Geometry check sheet. Reference: the model listing, model coordinates, mm. Face numbers are marked on the shaded views. A direction names the side the tool comes from. Round coordinates to 2 decimals unless told otherwise and drop trailing zeros. Order: outer loops, then holes, each group sorted by start corner. A loop starts at its lowest first (then second) coordinate and runs counter-clockwise, first axis right, second up.
(1) Set-up check for the marked faces 4, 5 and 6: record each of +Z, -Z, +X, -X, +Y, -Y from which the full face is reachable in a straight line by a thin tool's end or side.
(2) Thickness scan on L1, parallel to X at y = 16.5, z = 0.5; L2, parallel to Y at x = -12, z = 3 (3 decimals); L3, parallel to Y at x = 14, z = -3.5 (3 decimals). Record the ranges inside material, lowest first.
(3) Draft check along X on the marked faces 1, 2 and 3. Enter one of: pulls with the +X half, pulls with the -X half, needs draft (parallel to the pull), parting line crosses it, or undercut.
(4) Cross-section at C-C on z = -2.75. Enter the section's corners in (x, y) (3 decimals).
(5) Gauge pin test, flat ends, axial feed: P1, Ø5, axis at x = -12.5, y = 10.5, coming from the -Z side; P2, Ø3, axis at x = -1.5, z = -2, coming from the +Y side; P3, Ø4, axis at x = 14.5, z = 1, coming from the -Y side. Record the tip position at first contact, or that the pin passes through.
(6) Cross-section at A-A on z = 2. Enter the section's corners in (x, y) (3 decimals).
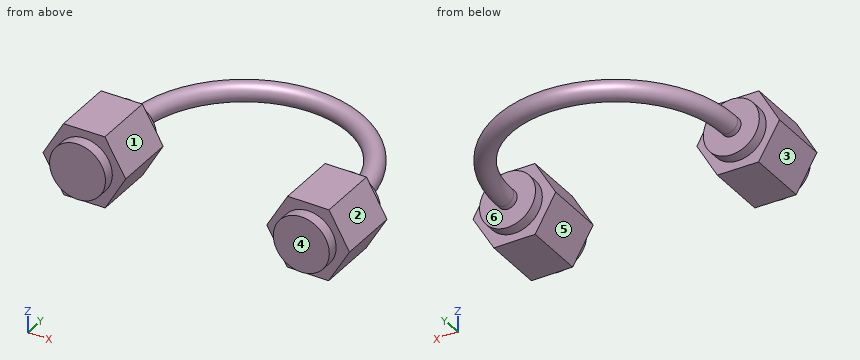
from build123d import *

# Parameters (mm, degrees)
SKETCH1_R             = 3.175
BOSS_EXTRUDE1_DEPTH   = 9.525
BOSS_EXTRUDE1_2_DEPTH = 9.525
BOSS_EXTRUDE2_START   = -1.27
BOSS_EXTRUDE2_DEPTH   = 6.985
SKETCH4_R             = 1.0922


with BuildPart() as part:
    # Sketch1 → Boss-Extrude1 (new body)
    with BuildSketch(Plane(origin=(0, 0, 0), x_dir=(1, 0, 0), z_dir=(0, 1, 0))):
        with Locations(Location((-12.7, 0, 0), (0, 0, 90))):
            Circle(SKETCH1_R)
    extrude(amount=BOSS_EXTRUDE1_DEPTH)

    # Sketch2 → Boss-Extrude2 (add)
    with BuildSketch(Plane(origin=(0, 9.525, 0), x_dir=(1, 0, 0), z_dir=(0, 1, 0)).offset(BOSS_EXTRUDE2_START)):
        Polygon((-8.007347217, -0.021706912), (-10.334874871, 4.053103065), (-15.027527654, 4.074809978), (-17.392652783, 0.021706912), (-15.065125129, -4.053103065), (-10.372472346, -4.074809978), align=None)
    boss_extrude2 = extrude(amount=-BOSS_EXTRUDE2_DEPTH)



with BuildPart() as body_2:
    # Sketch1 → Boss-Extrude1 2 (new body)
    with BuildSketch(Plane(origin=(0, 0, 0), x_dir=(1, 0, 0), z_dir=(0, 1, 0))):
        with Locations(Location((12.7, 0, 0), (0, 0, 90))):
            Circle(SKETCH1_R)
    extrude(amount=BOSS_EXTRUDE1_2_DEPTH)

    # Mirror1: Boss-Extrude2 across plane
    add(boss_extrude2.mirror(Plane(origin=(0, 0, 0), x_dir=(0, 0, 1), z_dir=(1, 0, 0))))


with BuildPart() as part_1:
    add(part.part)

    add(body_2.part)  # Sweep1 merges body 2
    # Sweep1: sweep along a path in Sketch3
    with BuildLine(Plane.XY) as sweep1_path:
        Line((-12.7, 9.525), (-12.7, 10.16))
        ThreePointArc((-12.7, 10.16), (0, 22.86), (12.7, 10.16))
        Line((12.7, 10.16), (12.7, 9.525))
    # Sketch4 → Sweep1 (sweep)
    with BuildSketch(Plane(origin=(0, 9.525, 0), x_dir=(1, 0, 0), z_dir=(0, 1, 0))):
        with Locations((-12.7, 0)):
            Circle(SKETCH4_R)
    sweep(path=sweep1_path.line)


solid = part_1.part
Found:
1. face 4: +Z, -Z, +X, -X, -Y
1. face 5: -Z, -Y
1. face 6: none
2. L1: x = -12.11 to -9.87, 9.87 to 12.11
2. L2: y = 0 to 9.525
2. L3: y = 1.27 to 8.255
3. face 1: undercut
3. face 2: pulls with the +X half
3. face 3: pulls with the -X half
4. outline: (-15.801, 1.27) - (-14.287, 1.27) - (-14.287, 0) - (-11.113, 0) - (-11.113, 1.27) - (-9.591, 1.27) - (-9.591, 8.255) - (-11.113, 8.255) - (-11.113, 9.525) - (-14.287, 9.525) - (-14.287, 8.255) - (-15.801, 8.255) - close; (9.591, 1.27) - (11.113, 1.27) - (11.113, 0) - (14.287, 0) - (14.287, 1.27) - (15.801, 1.27) - (15.801, 8.255) - (14.287, 8.255) - (14.287, 9.525) - (11.113, 9.525) - (11.113, 8.255) - (9.591, 8.255) - close
5. P1: stops at z = -4.07
5. P2: stops at y = 23.76
5. P3: stops at y = 0
6. outline: (-16.238, 1.27) - (-15.166, 1.27) - (-15.166, 0) - (-10.234, 0) - (-10.234, 1.27) - (-9.162, 1.27) - (-9.162, 8.255) - (-10.234, 8.255) - (-10.234, 9.525) - (-15.166, 9.525) - (-15.166, 8.255) - (-16.238, 8.255) - close; (9.162, 1.27) - (10.234, 1.27) - (10.234, 0) - (15.166, 0) - (15.166, 1.27) - (16.238, 1.27) - (16.238, 8.255) - (15.166, 8.255) - (15.166, 9.525) - (10.234, 9.525) - (10.234, 8.255) - (9.162, 8.255) - close
